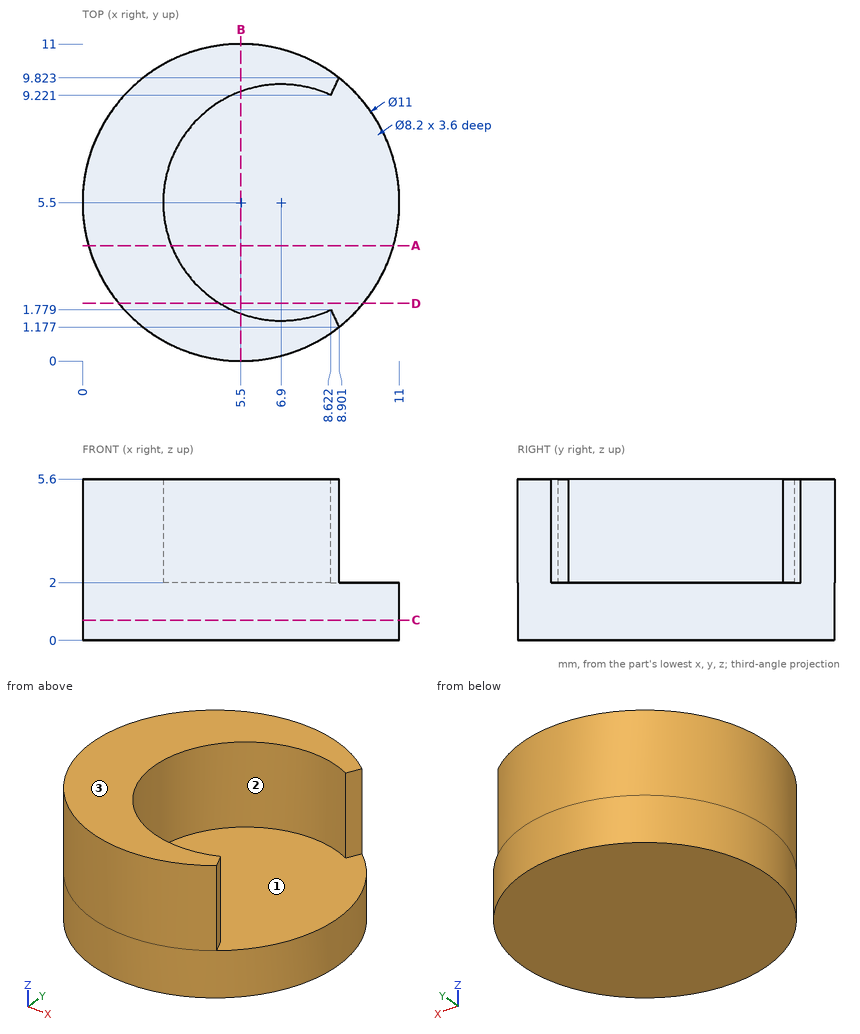
The drawing under review shows one solid part. Ordinate dimensions are in mm from its lowest x, y, z. Round coordinates to 2 decimals unless told otherwise and drop trailing zeros. Loops run counter-clockwise (first coordinate to the right, second up) from the corner with the lowest first, then second, coordinate; pieces in that order, holes last. Notation, with made-up numbers: (84, -16.5) - (108, -16.5) arc R21 cw to (108, 22.5) - close; hole circle Ø6 at (53.5, -33.75). An arc over 180 degrees is marked (long way). One line per question, with ' | ' between items.
Q1. Take a section at A-A (y = 4). Give the boundary of the cut face in (x, z).
Taken from the geometry:
outline: (0.21, 0) - (10.79, 0) - (10.79, 2) - (3.08, 2) - (3.08, 5.6) - (0.21, 5.6) - close
Q2. Take a section at C-C (z = 0.7). Give the boundary of the cut face in (x, y).
Taken from the geometry:
outline: circle Ø11 at (5.5, 5.5)
Q3. The part is to be moulded in two halves that separate along Y. For the marked faces 1, 2 and 3, say which applies: released by +Y, released by -Y, zero draft, split by the parting line, or undercut.
Taken from the geometry:
face 1: undercut | face 2: undercut | face 3: zero draft
Q4. Take a section at B-B (x = 5.5). Give the boundary of the cut face in (y, z).
Taken from the geometry:
outline: (0, 0) - (11, 0) - (11, 5.6) - (9.35, 5.6) - (9.35, 2) - (1.65, 2) - (1.65, 5.6) - (0, 5.6) - close
Q5. For pin 1 (4 mm diameter, centred on x = 7, y = 5, fed in from +Z); pin 2 (1.5 mm diameter, centred on y = 7.5, z = 2.5, fed in from +X); pin 3 (1.5 mm diameter, centred on y = 9, z = 0.5, fed in from +X), all flat-tipped, find the tip position at first contact; note any pin that passes through.
Taken from the geometry:
pin 1: stops at z = 2 | pin 2: stops at x = 10.81 | pin 3: stops at x = 10.26
Q6. Take a section at D-D (y = 2). Give the boundary of the cut face in (x, z) (1 decimal), and give its area (3 significant figures).
Taken from the geometry:
outline: (1.3, 0) - (9.7, 0) - (9.7, 2) - (4.8, 2) - (4.8, 5.6) - (1.3, 5.6) - close | area: 29.6 mm²
Q7. For line 1 along Z through (x, y) = (5, 5.75); line 2 along Y through (x, z) = (7.25, 2.1) (1 decimal); line 3 along Y through (x, z) = (6.9, 4.6), list the stretches that pass through material, from the lowest coordinate up. Write a range as [from, to].
Taken from the geometry:
line 1: z = [0, 2] | line 2: y = [0.3, 1.4], [9.6, 10.7] | line 3: y = [0.18, 1.4], [9.6, 10.82]
